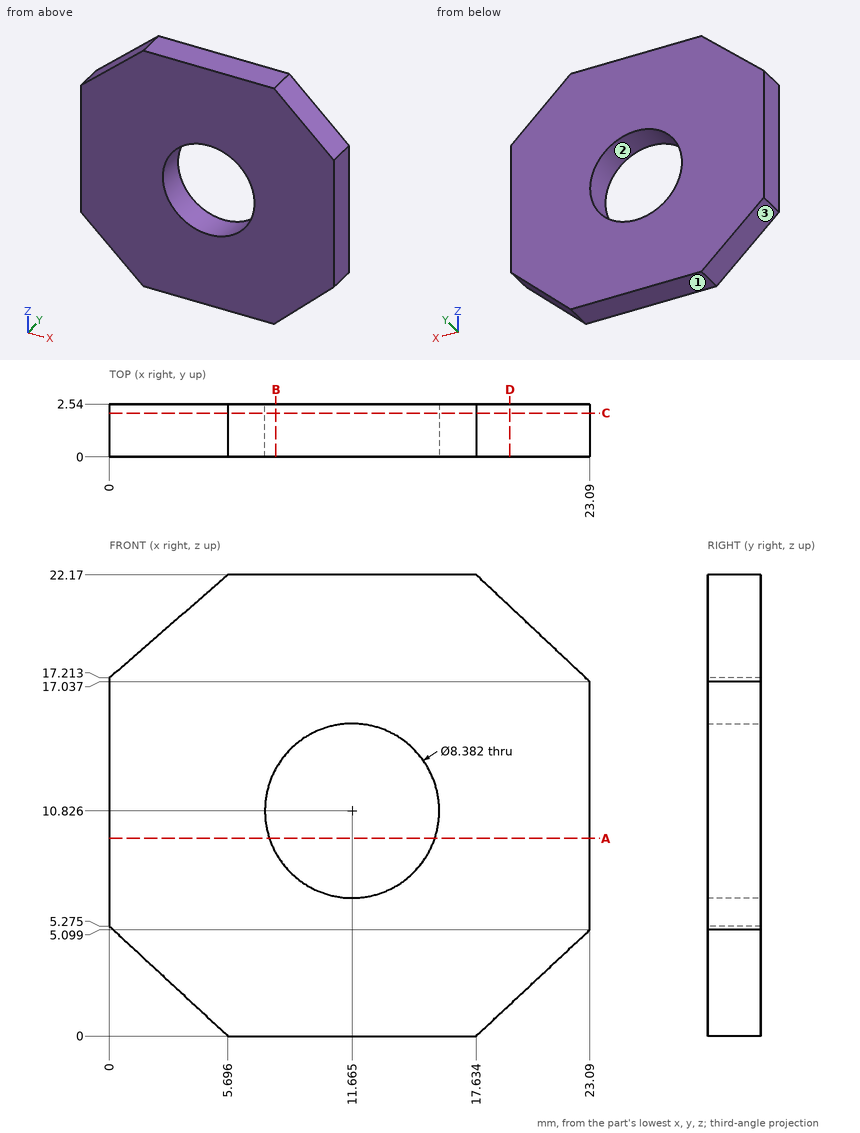
Could you check a few things on this drawing? It's one solid part, dimensions in mm from its lowest x, y, z. Coordinates: 2 decimals unless noted, no trailing zeros. Write each loop counter-clockwise with the first axis right and the second up, starting at its lowest first coordinate (ties: lowest second). Pieces come first, ordered by that corner, then holes. Notation, with made-up numbers: (83.25, -19) - (141.25, -19) arc R7 cw to (141.25, -12) - close; hole circle Ø4 at (74, -8). An arc over 180 degrees is marked (long way). Return JSON: item names as keys, results as strings. Group by question number.
Item 1: If we section it at B-B (x = 8): Write out the boundary of the cut face in (y, z).
Item 2: If we section it at A-A (z = 9.5): Write out the boundary of the cut face in (x, y).
Item 3: If we section it at C-C (y = 2.1): Write out the boundary of the cut face in (x, z) (1 decimal), then the cut area to 3 significant figures.
Item 4: If we section it at D-D (x = 19.25): Write out the boundary of the cut face in (y, z), then the cut area to 3 significant figures.
Item 5: Please list where these lines run through material, in increasing order: probe 1 along Z at (x, y) = (11.75, 1.45); probe 2 along X at (y, z) = (0.7, 10.75) (1 decimal); probe 3 along X at (y, z) = (0.4, 11.5).
Item 6: We'd pull the mould along X, two halves only. Please class the marked faces 1, 2 and 3: pulls with the +X half, pulls with the -X half, needs draft (parallel to the pull), parting line crosses it, or undercut.
Return value:
{
 "1": {"outline": "(0, 0) - (2.54, 0) - (2.54, 8.79) - (0, 8.79) - close; (0, 12.86) - (2.54, 12.86) - (2.54, 22.17) - (0, 22.17) - close"},
 "2": {"outline": "(0, 0) - (7.69, 0) - (7.69, 2.54) - (0, 2.54) - close; (15.64, 0) - (23.09, 0) - (23.09, 2.54) - (15.64, 2.54) - close"},
 "3": {"outline": "(0, 5.3) - (5.7, 0) - (17.6, 0) - (23.1, 5.1) - (23.1, 17) - (17.6, 22.2) - (5.7, 22.2) - (0, 17.2) - close; hole circle Ø8.4 at (11.7, 10.8)", "area": "400 mm^2"},
 "4": {"outline": "(0, 1.51) - (2.54, 1.51) - (2.54, 20.65) - (0, 20.65) - close", "area": "48.6 mm^2"},
 "5": {"probe 1": "z = 0 to 6.64, 15.02 to 22.17", "probe 2": "x = 0 to 7.5, 15.9 to 23.1", "probe 3": "x = 0 to 7.53, 15.8 to 23.09"},
 "6": {"face 1": "needs draft", "face 2": "undercut", "face 3": "pulls with the -X half"}
}
